Autodesk Inventor part; units mm, degrees
ref_plane "YZ Plane" through (0, 0, 0) normal (1, 0, 0) x (0, 1, 0)
ref_plane "XZ Plane" through (0, 0, 0) normal (0, 1, 0) x (-1, 0, 0)
ref_plane "XY Plane" through (0, 0, 0) normal (0, 0, 1) x (1, 0, 0)
sketch "Sketch1" plane through (0, 0, 0) normal (0, 0, 1) x (1, 0, 0)
  circle A0 centre (0, 0) radius 1.5
  circle A1 centre (0, 0) radius 2.75
  dimension "d0" = 3
  dimension "d3" = 5.5
extrude "Extrusion1" add sketch "Sketch1" along normal blind 16 contours A0
extrude "Extrusion2" add sketch "Sketch1" against normal blind 1.6 contours A0 | A1
sketch "Sketch2" plane through (0, 0, -1.6) normal (0, 0, -1) x (-1, 0, 0)
  circle A0 centre (0, 0) radius 1
  line L0 (0.5774, 1) -> (1.1547, 0)
  line L1 (1.1547, 0) -> (0.5774, -1)
  line L2 (0.5774, -1) -> (-0.5774, -1)
  line L3 (-0.5774, -1) -> (-1.1547, 0)
  line L4 (-1.1547, 0) -> (-0.5774, 1)
  line L5 (-0.5774, 1) -> (0.5774, 1)
  point P0 (0, 1)
  dimension "d6" = 2
extrude "Extrusion3" cut sketch "Sketch2" against normal blind 1
fillet "Fillet1" radius 1.35 1 edges at (-2.75, 0, -1.6)
thread "Thread1"
chamfer "Chamfer1" distance 0.2 angle 45 1 edges at (-1.5, 0, 16)
properties part number "COTS_GENERIC_M3x16_screw" material "Steel"
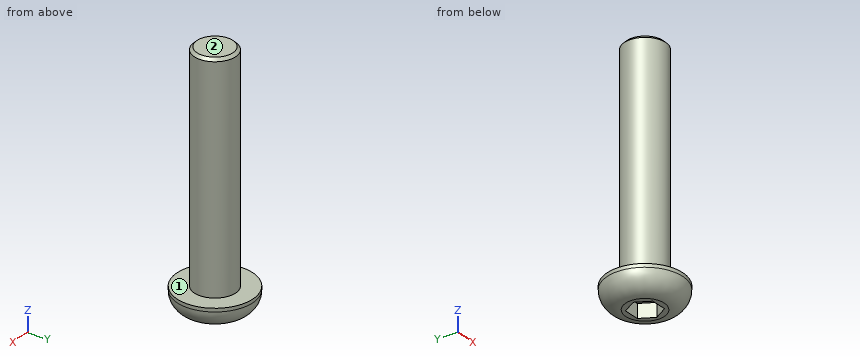
Can you work these out from the model? Positions are in its coordinate system, mm. Face numbers are marked on the shaded views. A direction names the side the tool comes from. Give positions to 0.01 mm unless a question says otherwise; leave off trailing zeros. Order: outer loops, then holes, each group sorted by start corner. A loop starts at its lowest first (then second) coordinate and runs counter-clockwise, first axis right, second up. Notation, with made-up numbers: (-5, -27.5) - (36, -27.5) arc R21 ccw to (36, -19.5) - close; hole circle Ø6 at (37, -19.75). An arc over 180 degrees is marked (long way). Use a Markdown table: item, result. Add a question column.
Q1. On a 3-axis mill with a long thin cutter (end or side, diameter ignored), from which of +Z, -Z, +X, -X, +Y, -Y can I reach the whole of each face in a straight line? I mean the marked faces 1 and 2. Say none if no direction works.
Q2. If we section it at B-B on z = 4: Write out the boundary of the cut face in (x, y), plus the area to 3 significant figures.
Q3. I'm going to push flat-ended pins straight in: pin 1 (1.5 mm diameter, centred on x = 1, z = 7.5, fed in from +Y); pin 2 (2 mm diameter, centred on y = 2, z = 3.5, fed in from +X); pin 3 (1.5 mm diameter, centred on y = -1.5, z = 8, fed in from +X). Where does each tip first touch, or does it pass through?
Q4. If we section it at A-A on x = 0: Write out the boundary of the cut face in (y, z), plus the area to 3 significant figures.
Q5. Please list where these lines run through material, in increasing order: line 1 along Z through (x, y) = (0.1, 0.15); line 2 along Z through (x, y) = (-1, -2.35); line 3 along Y through (x, z) = (0.7, 14.5).
Answers follow:
| question | item | result |
|---|---|---|
| 1 | face 1 | +Z |
| 1 | face 2 | +Z, +X, -X, +Y, -Y |
| 2 | outline | circle Ø3 at (0, 0) |
| 2 | area | 7.07 mm^2 |
| 3 | pin 1 | stops at y = 1.48 |
| 3 | pin 2 | stops at x = 1.12 |
| 3 | pin 3 | stops at x = 1.3 |
| 4 | outline | (-2.75, -0.25) arc R1.35 ccw to (-1.4, -1.6) - (-1, -1.6) - (-1, -0.6) - (1, -0.6) - (1, -1.6) - (1.4, -1.6) arc R1.35 ccw to (2.75, -0.25) - (2.75, 0) - (1.5, 0) - (1.5, 15.8) - (1.3, 16) - (-1.3, 16) - (-1.5, 15.8) - (-1.5, 0) - (-2.75, 0) - close |
| 4 | area | 54.0 mm^2 |
| 5 | line 1 | z = -0.6 to 16 |
| 5 | line 2 | z = -0.95 to 0 |
| 5 | line 3 | y = -1.33 to 1.33 |
